The listing builds one solid part. Answer for the finished solid, in the listing's coordinates (mm). A direction names the side the tool comes from. Give positions to 0.01 mm unless a question says otherwise; leave off trailing zeros. Loops run counter-clockwise (first coordinate to the right, second up) from the corner with the lowest first, then second, coordinate; pieces in that order, holes last. Notation, with made-up numbers: M -19,40.5 L 14,40.5 A6 ccw 14,50.5 Z; hole C 87.25,-22.75 d9. An arc over 180 degrees is marked long. One line per item, written item: value. Start each with the question number.
Q1. Flat-ended cylindrical pins translate along their axes: pin 1 (2 mm diameter, centred on x = -17, z = 1.5, fed in from -Y); pin 2 (4 mm diameter, centred on x = -18, y = -6.5, fed in from -Z); pin 3 (1 mm diameter, centred on y = -8.5, z = 3.5, fed in from -X); pin 4 (2 mm diameter, centred on x = 20, z = 1.5, fed in from +Y). Find the tip coordinate at first contact, or state that the pin passes through.
Q2. A cutting plane is placed at B-B, the plane z = 3.9. Determine the outline of the cut face in (x, y), and give its area (3 significant figures).
Q3. A cutting plane is placed at A-A, the plane y = -1. Determine the outline of the cut face in (x, z), and give its area (3 significant figures).
Q4. Consider L1, parallel to X at y = -1, z = 3.1; L2, parallel to X at y = -0.75, z = 1.65; L3, parallel to X at y = -23, z = 2. Determine where each line is inside the solid, lowest interval first.
Q5. For faces 1 (the cylindrical face through (-0.519, -24.995, 2.169)), 2 (the flat face through (18, -2.2, 2)), 3 (the flat face through (-18, -2.2, 2)), determine the directions among +Z, -Z, +X, -X, +Y, -Y from which every point of the face is accessible in a straight line to the end or side of a thin tool.
Q6. A cutting plane is placed at D-D, the plane y = -6. Determine the outline of the cut face in (x, z).
Q7. A cutting plane is placed at C-C, the plane x = -21. Determine the outline of the cut face in (y, z).
from build123d import *

# Parameters (mm, degrees)
SKETCH1_R           = 25
SKETCH1_R_2         = 8
BASE_EXTRUDE_DEPTH  = 4.4
CUT_EXTRUDE1_DEPTH  = 5.4
BOSS_EXTRUDE1_DEPTH = 4.4


with BuildPart() as part:
    # Sketch1 → Base-Extrude (new body)
    with BuildSketch(Plane.XY):
        Circle(SKETCH1_R)
        Circle(SKETCH1_R_2, mode=Mode.SUBTRACT)
    extrude(amount=BASE_EXTRUDE_DEPTH)

    # Sketch2 → Cut-Extrude1 (cut, through all)
    with BuildSketch(Plane.XY.offset(4.4)):
        Polygon((-31.283198073, -2.2), (32.499555714, -2.2), (32.499555714, 32.618237466), (-31.739332188, 32.618237466), align=None)
    extrude(amount=-CUT_EXTRUDE1_DEPTH, mode=Mode.SUBTRACT)

    # Sketch3 → Boss-Extrude1 (add)
    with BuildSketch(Plane.XY.offset(4.4)):
        with BuildLine():
            Line((7.691553809, -2.2), (11.86423196, -2.2))
            ThreePointArc((11.86423196, -2.2), (9.256550998, -1.233150178), (7.909487973, 1.2))
            ThreePointArc((7.909487973, 1.2), (7.983616109, -0.511736089), (7.691553809, -2.2))
        make_face()
        with BuildLine():
            Line((-11.86423196, -2.2), (-7.691553809, -2.2))
            ThreePointArc((-7.691553809, -2.2), (-7.983616109, -0.511736089), (-7.909487973, 1.2))
            ThreePointArc((-7.909487973, 1.2), (-9.256550998, -1.233150178), (-11.86423196, -2.2))
        make_face()
    extrude(amount=-BOSS_EXTRUDE1_DEPTH)


solid = part.part
Answer block:
1. pin 1: y = -19.21
1. pin 2: z = 0
1. pin 3: x = -23.69
1. pin 4: y = -2.2
2. outline: M -24.9,-2.2 A25 ccw 24.9,-2.2 L 11.86,-2.2 A4 cw 7.91,1.2 A8 cw long -7.91,1.2 A4 cw -11.86,-2.2 Z
2. area: 813 mm^2
3. outline: M -9.01,0 L -7.94,0 L -7.94,4.4 L -9.01,4.4 Z; M 7.94,0 L 9.01,0 L 9.01,4.4 L 7.94,4.4 Z
3. area: 9.42 mm^2
4. L1: -9.01 to -7.94, 7.94 to 9.01
4. L2: -8.78 to -7.96, 7.96 to 8.78
4. L3: -9.8 to 9.8
5. face 1: +Z, -Z, -Y
5. face 2: +Z, -Z, +X, +Y
5. face 3: +Z, -Z, -X, +Y
6. outline: M -24.27,0 L -5.29,0 L -5.29,4.4 L -24.27,4.4 Z; M 5.29,0 L 24.27,0 L 24.27,4.4 L 5.29,4.4 Z
7. outline: M -13.56,0 L -2.2,0 L -2.2,4.4 L -13.56,4.4 Z
